Input: part model. Units: mm. Frame: model coordinates. A direction names the side the tool comes from. Round coordinates to 2 decimals unless told otherwise and drop trailing zeros. Write each loop counter-clockwise with the first axis right and the second up, starting at its lowest first coordinate (ties: lowest second). Pieces come first, ordered by that corner, then holes. Notation, with made-up numbers: (-32.75, 37) - (10.25, 37) arc R10 ccw to (10.25, 42) - close; hole circle Ø3 at (70, 88). An arc over 180 degrees is marked (long way). Use one line per item in the form item = value.
```python
from build123d import *

# Parameters (mm, degrees)
SKETCH_W        = 19
SKETCH_H        = 12
SKETCH_R        = 1.6
SKETCH_R_2      = 1.5
PAD_DEPTH       = 5
SKETCH001_W     = 14
SKETCH001_H     = 12
SKETCH001_R     = 2.5
SKETCH001_R_2   = 1
POCKET_DEPTH    = 3.001
POCKET001_DEPTH = 2.001
FILLET_R        = 3


with BuildPart() as part:
    # Sketch → Pad (new body)
    with BuildSketch(Plane.XY):
        with Locations((9.5, 6)):
            Rectangle(SKETCH_W, SKETCH_H)
        with Locations((2, 6)):
            Circle(SKETCH_R, mode=Mode.SUBTRACT)
        with Locations((9, 6)):
            Circle(SKETCH_R_2, mode=Mode.SUBTRACT)
    extrude(amount=PAD_DEPTH)

    # Sketch001 (on DatumPlane) → Pocket (cut, through all)
    with BuildSketch(Plane.XY.offset(2)):
        with Locations((12, 6)):
            Rectangle(SKETCH001_W, SKETCH001_H)
        with Locations((9, 6)):
            Circle(SKETCH001_R, mode=Mode.SUBTRACT)
        with Locations((14, 9.1)):
            Circle(SKETCH001_R_2, mode=Mode.SUBTRACT)
        with Locations((14, 2.9)):
            Circle(SKETCH001_R_2, mode=Mode.SUBTRACT)
    extrude(amount=POCKET_DEPTH, mode=Mode.SUBTRACT)

    # Sketch002 (on DatumPlane) → Pocket001 (cut, through all)
    with BuildSketch(Plane.XY.offset(2)):
        Polygon((4.9, 4.325684), (4.9, 7.674316), (2, 9.348632), (-0.9, 7.674316), (-0.9, 4.325684), (2, 2.651368), align=None)
    extrude(amount=-POCKET001_DEPTH, mode=Mode.SUBTRACT)

    # Fillet
    fillet_edges = [part.edges().sort_by_distance(p)[0] for p in [
        (19, 0, 1),
        (19, 12, 1),
    ]]
    fillet(fillet_edges, radius=FILLET_R)


solid = part.part
```
(1) Cut plane B-B on x = 9. Output: boundary loops of the cut face in (y, z), then the cut area to 3 significant figures.
Derived:
outline = (0, 0) - (4.5, 0) - (4.5, 5) - (3.5, 5) - (3.5, 2) - (0, 2) - close; (7.5, 0) - (12, 0) - (12, 2) - (8.5, 2) - (8.5, 5) - (7.5, 5) - close
area = 24.0 mm^2
(2) Cut plane A-A on z = 4.25. Output: boundary loops of the cut face in (x, y).
Derived:
outline = (0, 0) - (5, 0) - (5, 12) - (0, 12) - close; circle Ø5 at (9, 6); circle Ø2 at (14, 2.9); circle Ø2 at (14, 9.1); hole circle Ø3.2 at (2, 6); hole circle Ø3 at (9, 6)
(3) First-contact query: pin 1 Ø0.9 at (y, z) = (7.5, 3) entering from +X; pin 2 Ø1.5 at (x, y) = (2.5, 5.5) entering from -Z; pin 3 Ø1.5 at (y, z) = (5.5, 1) entering from -X; pin 4 Ø5 at (x, y) = (2, 6) entering from +Z. Flat tips, straight axial feed; report the tip coordinate or a pass-through.
Derived:
pin_1 = 11.27
pin_2 = through
pin_3 = 4.9
pin_4 = 5
(4) Cut plane C-C on y = 6. Output: boundary loops of the cut face in (x, z), then the cut area to 3 significant figures.
Derived:
outline = (0, 2) - (0.4, 2) - (0.4, 5) - (0, 5) - close; (3.6, 2) - (4.9, 2) - (4.9, 0) - (7.5, 0) - (7.5, 5) - (6.5, 5) - (6.5, 2) - (5, 2) - (5, 5) - (3.6, 5) - close; (10.5, 0) - (19, 0) - (19, 2) - (11.5, 2) - (11.5, 5) - (10.5, 5) - close
area = 33.6 mm^2
(5) Material intervals for L1, parallel to Y at x = 2, z = 3.15; L2, parallel to X at y = 3, z = 2.1; L3, parallel to Z at x = 18, y = 10, sorted ascending.
Derived:
L1 = 0 to 4.4, 7.6 to 12
L2 = 0 to 5, 13.01 to 14.99
L3 = 0 to 2
(6) Access query for faces 4 (the face through (6, 0, 1)), 5 (the face through (14.924, 2.517, 3.479)), 6 (the face through (1.014, 8.779, 1.014)), 7 (the face through (5, 6, 3)), 8 (the face through (6, 12, 1)). Directions: +Z, -Z, +X, -X, +Y, -Y. A direction counts if a zero-diameter tool reaches every point of the face in a straight line with its end or side. Return the directions, or none.
Derived:
face_4 = +Z, -Z, +X, -X, -Y
face_5 = +Z
face_6 = -Z
face_7 = +Z, +Y, -Y
face_8 = +Z, -Z, +X, -X, +Y
(7) Cut plane D-D on z = 1.65. Output: boundary loops of the cut face in (x, y), then the cut area to 3 significant figures.
Derived:
outline = (0, 0) - (16, 0) arc R3 ccw to (19, 3) - (19, 9) arc R3 ccw to (16, 12) - (0, 12) - (0, 8.19) - (2, 9.35) - (4.9, 7.67) - (4.9, 4.33) - (2, 2.65) - (0, 3.81) - close; hole circle Ø3 at (9, 6)
area = 191 mm^2
(8) Draft query along X for faces 1 (the face through (14, 9, 5)), 2 (the face through (0, 5.9, 2.5)), 3 (the face through (3.47, 8.5, 1.01)). Return one class per face: released by +X, released by -X, zero draft, split by the parting line, or undercut.
Derived:
face_1 = zero draft
face_2 = released by -X
face_3 = undercut
